Design review of the part built by this model. Coordinates are the model's own, in mm. A direction names the side the tool comes from. Give positions to 0.01 mm unless a question says otherwise; leave off trailing zeros. Loops run counter-clockwise (first coordinate to the right, second up) from the corner with the lowest first, then second, coordinate; pieces in that order, holes last. Notation, with made-up numbers: (3, 18) - (59, 18) arc R15 ccw to (59, 32) - close; hole circle Ø9 at (84, 6.5). An arc over 180 degrees is marked (long way). One line per item, written item: value. Start each with the question number.
```python
from build123d import *

# Parameters (mm, degrees)
SKETCH_11_W         = 15
SKETCH_11_H         = 15
SKETCH_11_W_2       = 13
SKETCH_11_H_2       = 13
F_15X15X1_1_DEPTH   = 210
SKETCH_12_R         = 1.45
CUT_EXTRUDE_1_DEPTH = 107.330851591
SKETCH_14_R         = 1.45
CUT_EXTRUDE_3_DEPTH = 107.330851591
SKETCH_15_R         = 1.45
CUT_EXTRUDE_4_DEPTH = 107.330851591


with BuildPart() as part:
    # 草图11 → 铝管 15X15X1(1) (new body)
    with BuildSketch(Plane(origin=(-105, 0, 0), x_dir=(0, 0, -1), z_dir=(1, 0, 0))):
        Rectangle(SKETCH_11_W, SKETCH_11_H)
        Rectangle(SKETCH_11_W_2, SKETCH_11_H_2, mode=Mode.SUBTRACT)
    extrude(amount=F_15X15X1_1_DEPTH)

    # 草图12 → 切除-拉伸1 (cut, through all)
    with BuildSketch(Plane(origin=(0, 0, -7.5), x_dir=(-1, 0, 0), z_dir=(0, 0, -1))):
        with Locations((22.5, 0)):
            Circle(SKETCH_12_R)
        with Locations((65, 0)):
            Circle(SKETCH_12_R)
        with Locations((-65, 0)):
            Circle(SKETCH_12_R)
        with Locations((-22.5, 0)):
            Circle(SKETCH_12_R)
    extrude(amount=-CUT_EXTRUDE_1_DEPTH, mode=Mode.SUBTRACT)

    # 草图14 → 切除-拉伸3 (cut, through all)
    with BuildSketch(Plane(origin=(0, 7.5, 0), x_dir=(1, 0, 0), z_dir=(0, 1, 0))):
        with Locations(Location((0, 0, 0), (0, 0, 270))):
            Circle(SKETCH_14_R)
        with Locations(Location((45, 0, 0), (0, 0, 270))):
            Circle(SKETCH_14_R)
        with Locations(Location((-45, 0, 0), (0, 0, 90))):
            Circle(SKETCH_14_R)
    extrude(amount=-CUT_EXTRUDE_3_DEPTH, mode=Mode.SUBTRACT)

    # 草图15 → 切除-拉伸4 (cut, through all)
    with BuildSketch(Plane.XZ.offset(7.5)):
        with Locations(Location((-97.5, 0, 0), (0, 0, 270))):
            Circle(SKETCH_15_R)
        with Locations(Location((97.5, 0, 0), (0, 0, 270))):
            Circle(SKETCH_15_R)
    extrude(amount=-CUT_EXTRUDE_4_DEPTH, mode=Mode.SUBTRACT)


solid = part.part
```
(1) Machinability: for faces 5 (the flat face through (-1, 6.5, 2)), 6 (the flat face through (-1, 7.5, 2)), which of the approach directions +Z, -Z, +X, -X, +Y, -Y give a long, thin tool a straight path to every point of the face, cutting with its end or side? Answer none if there is none.
(2) Take a section at A-A on z = -4.25. State the section outline as (x, y) points.
(3) Take a section at B-B on x = -71.5. State the section outline as (y, z) points.
(4) To check wall thickness, follow L1, parallel to X at y = -7.15, z = 0; L2, parallel to Z at x = -72, y = 1.25. State the ranges of each line that lie inside material, in increasing order. Write a range as from..to.
(5) Draft analysis for pull direction Z (two halves, no side actions). For faces 1 (the flat face through (-105, 0, 7)), 2 (the flat face through (-1, 0, -7.5)), 3 (the flat face through (-1, -6.5, 2)), 4 (the flat face through (-1, 0, -6.5)), state which applies: pulls with the +Z half, pulls with the -Z half, needs draft (parallel to the pull), parting line crosses it, or undercut.
Here are the results:
1. face 5: +X, -X
1. face 6: +Z, -Z, +X, -X, +Y
2. outline: (-105, -7.5) - (105, -7.5) - (105, -6.5) - (-105, -6.5) - close; (-105, 6.5) - (105, 6.5) - (105, 7.5) - (-105, 7.5) - close
3. outline: (-7.5, -7.5) - (7.5, -7.5) - (7.5, 7.5) - (-7.5, 7.5) - close; hole (-6.5, -6.5) - (6.5, -6.5) - (6.5, 6.5) - (-6.5, 6.5) - close
4. L1: -105..-98.95, -96.05..-46.45, -43.55..-1.45, 1.45..43.55, 46.45..96.05, 98.95..105
4. L2: -7.5..-6.5, 6.5..7.5
5. face 1: needs draft
5. face 2: pulls with the -Z half
5. face 3: undercut
5. face 4: undercut
